Job drawing, mm, ordinate dimensions from the low corner. One solid piece. A direction names the side the tool comes from. Give positions to 0.01 mm unless a question says otherwise; leave off trailing zeros. Loops run counter-clockwise (first coordinate to the right, second up) from the corner with the lowest first, then second, coordinate; pieces in that order, holes last. Notation, with made-up numbers: (41.25, -25) -> (72.25, -25) arc R22 cw to (72.25, -2) -> close; hole circle Ø7 at (-13, -15.75). An arc over 180 degrees is marked (long way). Answer as a JSON object with one key per item and string values. Group by question number.
Q1. Tool access for the marked faces 1, 2 and 3: list every direction of +Z, -Z, +X, -X, +Y, -Y with a clear straight run to the whole face (end or side of a thin tool).
Q2. Band-saw the part on C-C, the plane x = 170. Write the cut outline in (y, z), plus the area to 3 significant figures.
Q3. Band-saw the part on A-A, the plane z = 17. Write the cut outline in (x, y).
Q4. Drop flat-ended pins along their axis: pin 1 (11 mm diameter, centred on x = 8.5, z = 74.5, fed in from -Y); pin 2 (8 mm diameter, centred on x = 6, y = 122, fed in from +Z); pin 3 (3 mm diameter, centred on x = 35, z = 46, fed in from +Y); pin 4 (21 mm diameter, centred on y = 86, z = 52, fed in from +X). Give the stop position or say it passes through.
Q5. Two-plate mould, pull along X, no slides. Class the marked faces 4, 5 and 6: pulls with the +X half, pulls with the -X half, needs draft (parallel to the pull), parting line crosses it, or undercut.
Q6. Band-saw the part on B-B, the plane y = 112. Write the cut outline in (x, z), plus the area to 3 significant figures.
Q7. Band-saw the part on D-D, the plane z = 45.5. Write the cut outline in (x, y), plus the area to 3 significant figures.
Q8. Wall check: probe 1 along X at (y, z) = (206.5, 32); probe 2 along Y at (x, z) = (170, 8.5); probe 3 along X at (y, z) = (203, 85). Give the ranges that are in metal, low to high. Write a range as from..to.
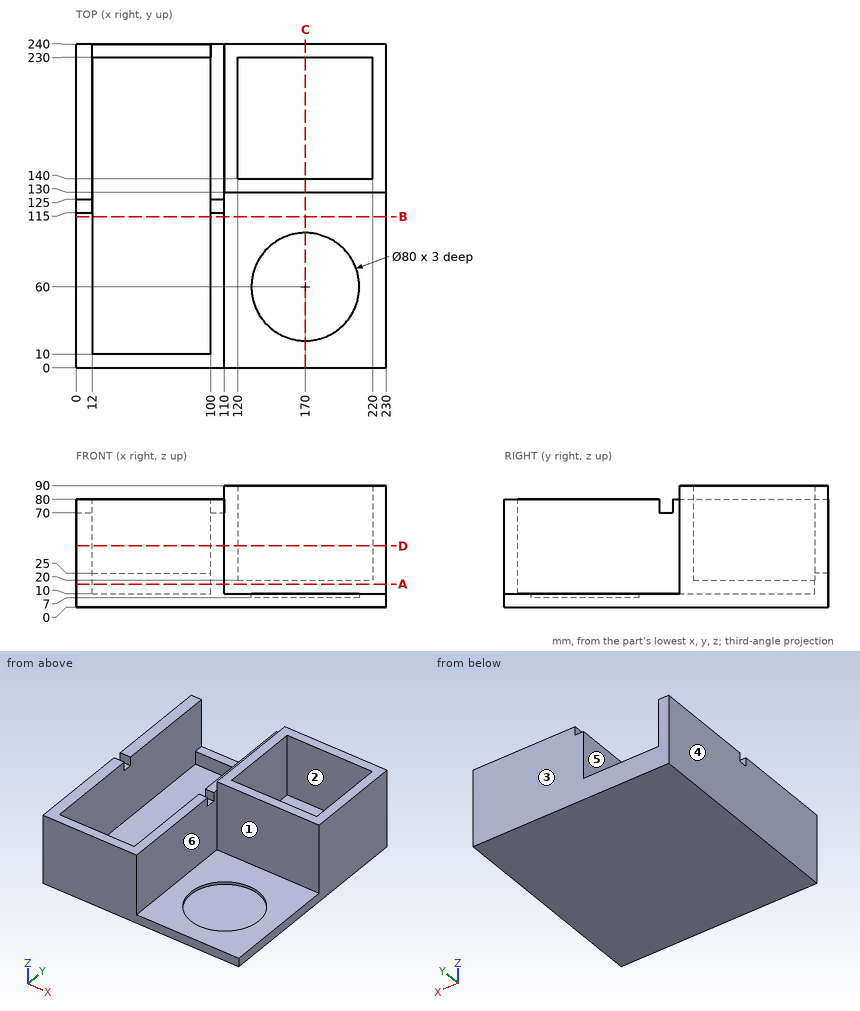
Worked answers:
{
 "1": {"face 1": "+Z, +X, -Y", "face 2": "+Z", "face 3": "+Z, -Z, +X, -X, +Y"},
 "2": {"outline": "(0, 0) -> (240, 0) -> (240, 90) -> (230, 90) -> (230, 20) -> (140, 20) -> (140, 90) -> (130, 90) -> (130, 10) -> (100, 10) -> (100, 7) -> (20, 7) -> (20, 10) -> (0, 10) -> close", "area": "4,660 mm2"},
 "3": {"outline": "(0, 0) -> (110, 0) -> (110, 130) -> (230, 130) -> (230, 240) -> (0, 240) -> close; hole (12, 10) -> (100, 10) -> (100, 230) -> (12, 230) -> close"},
 "4": {"pin 1": "y = 0", "pin 2": "z = 80", "pin 3": "y = 10", "pin 4": "x = 110"},
 "5": {"face 4": "pulls with the -X half", "face 5": "undercut", "face 6": "pulls with the +X half"},
 "6": {"outline": "(0, 0) -> (230, 0) -> (230, 10) -> (110, 10) -> (110, 80) -> (100, 80) -> (100, 10) -> (12, 10) -> (12, 80) -> (0, 80) -> close", "area": "3,840 mm2"},
 "7": {"outline": "(0, 0) -> (110, 0) -> (110, 130) -> (230, 130) -> (230, 240) -> (100, 240) -> (100, 10) -> (12, 10) -> (12, 240) -> (0, 240) -> close; hole (120, 140) -> (220, 140) -> (220, 230) -> (120, 230) -> close", "area": "10,400 mm2"},
 "8": {"probe 1": "0..12, 100..120, 220..230", "probe 2": "0..20, 100..240", "probe 3": "110..120, 220..230"}
}
